from build123d import *

# Parameters (mm, degrees)
F1_DEPTH  = 100
F3_DEPTH  = 70
F4_R      = 8.1
F4_R_2    = 3.1
F5_DEPTH  = 4.1237650092
F6_R      = 8.1
F6_R_2    = 3.1
F7_DEPTH  = 4.1237650092
F8_R      = 8.1
F8_R_2    = 3.1
F9_DEPTH  = 4.1237650092
F10_R     = 8.1
F10_R_2   = 3.1
F11_DEPTH = 4.1237650092
F12_R     = 3.05
F13_DEPTH = 5.1525521704
F14_R     = 3.05
F15_DEPTH = 5.1525521704
F16_R     = 3.05
F17_DEPTH = 5.1525521704
F18_R     = 3.05
F19_DEPTH = 5.1525521704


with BuildPart() as f1:
    # F0 (on Top) → F1 (new body)
    with BuildSketch(Plane.XY):
        with BuildLine():
            Line((17.5, 72.9297607291), (-17.5, 72.9297607291))
            ThreePointArc((-17.5, 72.9297607291), (-53.033008589, 53.033008589), (-72.9297607291, 17.5))
            Line((-72.9297607291, 17.5), (-72.9297607291, -17.5))
            ThreePointArc((-72.9297607291, -17.5), (-53.033008589, -53.033008589), (-17.5, -72.9297607291))
            Line((-17.5, -72.9297607291), (17.5, -72.9297607291))
            ThreePointArc((17.5, -72.9297607291), (53.033008589, -53.033008589), (72.9297607291, -17.5))
            Line((72.9297607291, -17.5), (72.9297607291, 17.5))
            ThreePointArc((72.9297607291, 17.5), (53.033008589, 53.033008589), (17.5, 72.9297607291))
        make_face()
        with BuildLine():
            ThreePointArc((-67.7772085586, 17.5), (-49.4974746831, 49.4974746831), (-17.5, 67.7772085586))
            Line((-17.5, 67.7772085586), (17.5, 67.7772085586))
            ThreePointArc((17.5, 67.7772085586), (49.4974746831, 49.4974746831), (67.7772085586, 17.5))
            Line((67.7772085586, 17.5), (67.7772085586, -17.5))
            ThreePointArc((67.7772085586, -17.5), (49.4974746831, -49.4974746831), (17.5, -67.7772085586))
            Line((17.5, -67.7772085586), (-17.5, -67.7772085586))
            ThreePointArc((-17.5, -67.7772085586), (-49.4974746831, -49.4974746831), (-67.7772085586, -17.5))
            Line((-67.7772085586, -17.5), (-67.7772085586, 17.5))
        make_face(mode=Mode.SUBTRACT)
    extrude(amount=F1_DEPTH)

    # F2 (on face) → F3 (join)
    with BuildSketch(Plane.XY.offset(100)):
        with BuildLine():
            Line((17.5, 71.9009735678), (-17.5, 71.9009735678))
            ThreePointArc((-17.5, 71.9009735678), (-52.3259018078, 52.3259018078), (-71.9009735678, 17.5))
            Line((-71.9009735678, 17.5), (-71.9009735678, -17.5))
            ThreePointArc((-71.9009735678, -17.5), (-52.3259018078, -52.3259018078), (-17.5, -71.9009735678))
            Line((-17.5, -71.9009735678), (17.5, -71.9009735678))
            ThreePointArc((17.5, -71.9009735678), (52.3259018078, -52.3259018078), (71.9009735678, -17.5))
            Line((71.9009735678, -17.5), (71.9009735678, 17.5))
            ThreePointArc((71.9009735678, 17.5), (52.3259018078, 52.3259018078), (17.5, 71.9009735678))
        make_face()
        with BuildLine():
            ThreePointArc((-67.7772085586, 17.5), (-49.4974746831, 49.4974746831), (-17.5, 67.7772085586))
            Line((-17.5, 67.7772085586), (17.5, 67.7772085586))
            ThreePointArc((17.5, 67.7772085586), (49.4974746831, 49.4974746831), (67.7772085586, 17.5))
            Line((67.7772085586, 17.5), (67.7772085586, -17.5))
            ThreePointArc((67.7772085586, -17.5), (49.4974746831, -49.4974746831), (17.5, -67.7772085586))
            Line((17.5, -67.7772085586), (-17.5, -67.7772085586))
            ThreePointArc((-17.5, -67.7772085586), (-49.4974746831, -49.4974746831), (-67.7772085586, -17.5))
            Line((-67.7772085586, -17.5), (-67.7772085586, 17.5))
        make_face(mode=Mode.SUBTRACT)
    extrude(amount=F3_DEPTH)

    # F4 (on face) → F5 (cut, through all)
    with BuildSketch(Plane.XZ.offset(71.9009735678)):
        with Locations((0, 153)):
            Circle(F4_R)
        with Locations((0, 134)):
            Circle(F4_R_2)
        with Locations((0, 117)):
            Circle(F4_R_2)
    extrude(amount=-F5_DEPTH, mode=Mode.SUBTRACT)

    # F6 (on face) → F7 (cut, through all)
    with BuildSketch(Plane.YZ.offset(71.9009735678)):
        with Locations((0, 153)):
            Circle(F6_R)
        with Locations((0, 134)):
            Circle(F6_R_2)
        with Locations((0, 117)):
            Circle(F6_R_2)
    extrude(amount=-F7_DEPTH, mode=Mode.SUBTRACT)

    # F8 (on face) → F9 (cut, through all)
    with BuildSketch(Plane(origin=(0, 71.9009735678, 0), x_dir=(-1, 0, 0), z_dir=(0, 1, 0))):
        with Locations((0, 153)):
            Circle(F8_R)
        with Locations((0, 134)):
            Circle(F8_R_2)
        with Locations((0, 117)):
            Circle(F8_R_2)
    extrude(amount=-F9_DEPTH, mode=Mode.SUBTRACT)

    # F10 (on face) → F11 (cut, through all)
    with BuildSketch(Plane(origin=(-71.9009735678, 0, 0), x_dir=(0, -1, 0), z_dir=(-1, 0, 0))):
        with Locations((0, 153)):
            Circle(F10_R)
        with Locations((0, 134)):
            Circle(F10_R_2)
        with Locations((0, 117)):
            Circle(F10_R_2)
    extrude(amount=-F11_DEPTH, mode=Mode.SUBTRACT)

    # F12 (on face) → F13 (cut, through all)
    with BuildSketch(Plane.YZ.offset(72.9297607291)):
        with Locations((0, 65)):
            Circle(F12_R)
        with Locations((0, 30)):
            Circle(F12_R)
    extrude(amount=-F13_DEPTH, mode=Mode.SUBTRACT)

    # F14 (on face) → F15 (cut, through all)
    with BuildSketch(Plane.XZ.offset(72.9297607291)):
        with Locations((0, 65)):
            Circle(F14_R)
        with Locations((0, 30)):
            Circle(F14_R)
    extrude(amount=-F15_DEPTH, mode=Mode.SUBTRACT)

    # F16 (on face) → F17 (cut, through all)
    with BuildSketch(Plane(origin=(0, 72.9297607291, 0), x_dir=(-1, 0, 0), z_dir=(0, 1, 0))):
        with Locations((0, 65)):
            Circle(F16_R)
        with Locations((0, 30)):
            Circle(F16_R)
    extrude(amount=-F17_DEPTH, mode=Mode.SUBTRACT)

    # F18 (on face) → F19 (cut, through all)
    with BuildSketch(Plane(origin=(-72.9297607291, 0, 0), x_dir=(0, -1, 0), z_dir=(-1, 0, 0))):
        with Locations((0, 65)):
            Circle(F18_R)
        with Locations((0, 30)):
            Circle(F18_R)
    extrude(amount=-F19_DEPTH, mode=Mode.SUBTRACT)


solid = f1.part
Geometry check sheet. Reference: the model listing, model coordinates, mm. A direction names the side the tool comes from. Round coordinates to 2 decimals unless told otherwise and drop trailing zeros. Write each loop counter-clockwise with the first axis right and the second up, starting at its lowest first coordinate (ties: lowest second). Pieces come first, ordered by that corner, then holes. Notation, with made-up numbers: (-9.5, 48.25) - (32.5, 48.25) arc R14 ccw to (32.5, 70.25) - close; hole circle Ø5 at (-22.5, 74.25). An arc over 180 degrees is marked (long way). One line per item, written item: value.
1. Cross-section at A-A on x = 13. Record the boundary of the cut face in (y, z), and give its area (3 significant figures).
The answers:
outline: (-72.93, 0) - (-67.78, 0) - (-67.78, 170) - (-71.9, 170) - (-71.9, 100) - (-72.93, 100) - close; (67.78, 0) - (72.93, 0) - (72.93, 100) - (71.9, 100) - (71.9, 170) - (67.78, 170) - close
area: 1,610 mm^2
2. Cross-section at C-C on z = 30. Give the number of separate pieces and of enclosed holes in the cut face, and give its area (3 significant figures).
The answers:
separate pieces: 4
enclosed holes: 0
area: 2,170 mm^2
3. Scan lines: L1, parallel to Z at x = 0, y = -71; L2, parallel to Y at x = -11.5, z = 18; L3, parallel to X at y = -3.5, z = 132.5. Record each from-to range of solid material in increasing order.
The answers:
L1: z = 0 to 26.95, 33.05 to 61.95, 68.05 to 113.9, 120.1 to 130.9, 137.1 to 144.9, 161.1 to 170
L2: y = -72.93 to -67.78, 67.78 to 72.93
L3: x = -71.9 to -67.78, 67.78 to 71.9
4. Cross-section at B-B on z = 107.5. Record the boundary of the cut face in (x, y).
The answers:
outline: (-71.9, -17.5) arc R74 ccw to (-17.5, -71.9) - (17.5, -71.9) arc R74 ccw to (71.9, -17.5) - (71.9, 17.5) arc R74 ccw to (17.5, 71.9) - (-17.5, 71.9) arc R74 ccw to (-71.9, 17.5) - close; hole (-67.78, -17.5) arc R70 ccw to (-17.5, -67.78) - (17.5, -67.78) arc R70 ccw to (67.78, -17.5) - (67.78, 17.5) arc R70 ccw to (17.5, 67.78) - (-17.5, 67.78) arc R70 ccw to (-67.78, 17.5) - close
5. Set-up check for faces 4 (the face through (-52.725, -51.924, 134.51)), 5 (the face through (0, 67.777, 84)), 6 (the face through (-71.901, 4, 135)): record each of +Z, -Z, +X, -X, +Y, -Y from which the full face is reachable in a straight line by a thin tool's end or side.
The answers:
face 4: +Z, -X, -Y
face 5: +Z, -Z
face 6: +Z, -X, +Y, -Y
6. Mould release check, pull along X, two halves, no side actions. Record for faces 1 (the face through (0, -70, 0)), 2 (the face through (-51.924, 52.725, 134.51)), 3 (the face through (0, -67.777, 84)): released by +X, released by -X, zero draft, split by the parting line, or undercut.
The answers:
face 1: zero draft
face 2: released by -X
face 3: undercut
7. Depth check by flat-ended pin: pin 1 Ø10 at (y, z) = (34, 38) entering from +X; pin 2 Ø9.5 at (x, z) = (0, 153) entering from -Y; pin 3 Ø21 at (y, z) = (0, 153) entering from -X; pin 4 Ø5 at (x, z) = (-52.5, 24) entering from -Y. Enter the tip coordinate at first touch or a pass-through.
The answers:
pin 1: stops at x = 69.17
pin 2: passes through
pin 3: stops at x = -71.9
pin 4: stops at y = -55.9
8. Cross-section at D-D on y = 39.5. Record the boundary of the cut face in (x, z).
The answers:
outline: (-63.76, 0) - (-57.79, 0) - (-57.79, 170) - (-62.58, 170) - (-62.58, 100) - (-63.76, 100) - close; (57.79, 0) - (63.76, 0) - (63.76, 100) - (62.58, 100) - (62.58, 170) - (57.79, 170) - close
